Input: part model. Units: mm. Frame: model coordinates. A direction names the side the tool comes from. Coordinates: 2 decimals unless noted, no trailing zeros. Order: outer loops, then holes, each group sorted by start corner. A loop starts at its lowest first (then second) coordinate and runs counter-clockwise, first axis right, second up.
from build123d import *

# Parameters (mm, degrees)
F0_R          = 120
F1_DEPTH      = 12
F1_DEPTH_BACK = 38
F2_R          = 110
F2_R_2        = 17.5
F3_DEPTH      = 38
F4_R          = 5
F5_R          = 15.2795
F6_DEPTH      = 15.2795
F8_R          = 120
F9_DEPTH      = 5
F10_R         = 12.5
F11_DEPTH     = 55.001
F12_R         = 120
F12_R_2       = 110
F13_DEPTH     = 3
F14_W         = 5
F14_H         = 122.5
F14_W_2       = 122.5
F14_H_2       = 5
F15_DEPTH     = 3
F16_R         = 136.7884680592
F16_R_2       = 100.9393969777
F17_DEPTH     = 5
F19_R         = 4
F20_DEPTH     = 25
F22_R         = 4
F23_DEPTH     = 25


# Not quite as in the source:
# - a fillet or chamfer that OpenCascade refuses, or shapes differently, is made with other operations: its cross-section is extruded or revolved along the edge and cut away or added


with BuildPart() as f1:
    # F0 (on Top) → F1 (new body, two sides)
    with BuildSketch(Plane.XY) as f1_sk:
        Circle(F0_R)
    extrude(amount=F1_DEPTH)
    extrude(f1_sk.sketch, amount=-F1_DEPTH_BACK)

    # F2 (on face) → F3 (cut)
    with BuildSketch(Plane(origin=(0, 0, -38), x_dir=(1, 0, 0), z_dir=(0, 0, -1))):
        Circle(F2_R)
        Circle(F2_R_2, mode=Mode.SUBTRACT)
    extrude(amount=-F3_DEPTH, mode=Mode.SUBTRACT)

    # F4
    f4_edges = [f1.edges().sort_by_distance(p)[0] for p in [
        (-17.5, 0, 0),
        (-110, 0, 0),
    ]]
    fillet(f4_edges, radius=F4_R)

    # F5 (on face) → F6 (cut)
    with BuildSketch(Plane(origin=(0, 0, 0), x_dir=(1, 0, 0), z_dir=(0, 0, -1))):
        with Locations((-60, 60)):
            Circle(F5_R)
        with Locations((-60, -60)):
            Circle(F5_R)
        with Locations((60, -60)):
            Circle(F5_R)
        with Locations((60, 60)):
            Circle(F5_R)
    extrude(amount=-F6_DEPTH, mode=Mode.SUBTRACT)

    # F8 (on face) → F9 (join)
    with BuildSketch(Plane.XY.offset(12)):
        Circle(F8_R)
    extrude(amount=F9_DEPTH)

    # F10 (on face) → F11 (cut, through all)
    with BuildSketch(Plane(origin=(0, 0, -38), x_dir=(1, 0, 0), z_dir=(0, 0, -1))):
        Circle(F10_R)
    extrude(amount=-F11_DEPTH, mode=Mode.SUBTRACT)

    # F12 (on face) → F13 (cut)
    with BuildSketch(Plane.XY.offset(17)):
        Circle(F12_R)
        Circle(F12_R_2, mode=Mode.SUBTRACT)
    extrude(amount=-F13_DEPTH, mode=Mode.SUBTRACT)

    # F14 (on face) → F15 (cut)
    with BuildSketch(Plane.XY.offset(17)):
        with Locations((0, -63.75)):
            Rectangle(F14_W, F14_H)
        with Locations((-63.75, 0)):
            Rectangle(F14_W_2, F14_H_2)
        Rectangle(F14_W, F14_H_2)
        with Locations((63.75, 0)):
            Rectangle(F14_W_2, F14_H_2)
        with Locations((0, 63.75)):
            Rectangle(F14_W, F14_H)
    extrude(amount=-F15_DEPTH, mode=Mode.SUBTRACT)

    # F16 (on face) → F17 (cut)
    with BuildSketch(Plane(origin=(0, 0, -38), x_dir=(1, 0, 0), z_dir=(0, 0, -1))):
        Circle(F16_R)
        Circle(F16_R_2, mode=Mode.SUBTRACT)
    extrude(amount=-F17_DEPTH, mode=Mode.SUBTRACT)

    # F18: fillet of radius 15.2795 on 4 edges, made by hand

    # F18_s1 → F18_t2 (revolve)
    with BuildSketch(Plane.XZ.offset(60)):
        with BuildLine():
            ThreePointArc((75.2795, 0), (69.9309062658, 8.6278977111), (60.3560955627, 12))
            Line((60.3560955627, 12), (75.2795, 12))
            Line((75.2795, 12), (75.2795, 0))
        make_face()
    revolve(axis=Axis((60, -60, 12), (0, 0, -1)))

    # F18_s3 → F18_t4 (revolve)
    with BuildSketch(Plane.XZ.offset(60)):
        with BuildLine():
            ThreePointArc((-44.7205, 0), (-50.0690937342, 8.6278977111), (-59.6439044373, 12))
            Line((-59.6439044373, 12), (-44.7205, 12))
            Line((-44.7205, 12), (-44.7205, 0))
        make_face()
    revolve(axis=Axis((-60, -60, 12), (0, 0, -1)))

    # F18_s5 → F18_t6 (revolve)
    with BuildSketch(Plane.XZ.offset(-60)):
        with BuildLine():
            ThreePointArc((-44.7205, 0), (-50.0690937342, 8.6278977111), (-59.6439044373, 12))
            Line((-59.6439044373, 12), (-44.7205, 12))
            Line((-44.7205, 12), (-44.7205, 0))
        make_face()
    revolve(axis=Axis((-60, 60, 12), (0, 0, -1)))

    # F18_s7 → F18_t8 (revolve)
    with BuildSketch(Plane.XZ.offset(-60)):
        with BuildLine():
            ThreePointArc((75.2795, 0), (69.9309062658, 8.6278977111), (60.3560955627, 12))
            Line((60.3560955627, 12), (75.2795, 12))
            Line((75.2795, 12), (75.2795, 0))
        make_face()
    revolve(axis=Axis((60, 60, 12), (0, 0, -1)))

    # F19 (on offset) → F20 (cut)
    with BuildSketch(Plane.XZ.offset(120)):
        with Locations((0, -19)):
            Circle(F19_R)
    extrude(amount=-F20_DEPTH, mode=Mode.SUBTRACT)

    # F22 (on offset) → F23 (cut)
    with BuildSketch(Plane.XZ.offset(-120)):
        with Locations((0, -19)):
            Circle(F22_R)
    extrude(amount=F23_DEPTH, mode=Mode.SUBTRACT)


solid = f1.part
Item 1: Pin query (flat end, axial travel): pin 1 Ø1.5 at (y, z) = (-47, -21) entering from -X; pin 2 Ø1.5 at (x, z) = (-74, 15.5) entering from +Y; pin 3 Ø8 at (x, y) = (-36, 85) entering from -Z; pin 4 Ø15 at (x, y) = (0, 0) entering from -Z. Return the tip coordinate at first contact, or that it passes through.
Response values:
pin 1: stops at x = -110.73
pin 2: stops at y = 82.06
pin 3: stops at z = 0
pin 4: passes through
Item 2: Cut plane A-A on z = -26.5. Return loops of the section in (x, y).
Response values:
outline: circle Ø240 at (0, 0); circle Ø35 at (0, 0); hole circle Ø220 at (0, 0); hole circle Ø25 at (0, 0)
Item 3: Draft query along X for faces 1 (the face through (-1, -25, 0)), 2 (the face through (-45, -44, 17)), 3 (the face through (-0.521, -115.033, -15.034)), 4 (the face through (-78.608, -76.947, 15.521)). Return one class per face: pulls with the +X half, pulls with the -X half, needs draft (parallel to the pull), parting line crosses it, or undercut.
Response values:
face 1: undercut
face 2: needs draft
face 3: undercut
face 4: pulls with the -X half
Item 4: Access query for faces 5 (the face through (-23.846, 107.384, -19.196)), 6 (the face through (78.608, 76.947, 15.521)), 7 (the face through (-76.947, 78.608, 15.521)). Directions: +Z, -Z, +X, -X, +Y, -Y. A direction counts if a zero-diameter tool reaches every point of the face in a straight line with its end or side. Return the directions, or none.
Response values:
face 5: -Z
face 6: +Z, +X, +Y
face 7: +Z, -X, +Y
Item 5: Ray query, probe 1 along Y at (x, z) = (0, -11.25); probe 2 along Z at (x, y) = (0, 113.25). Return the intervals inside material, ascending.
Response values:
probe 1: y = -120 to -110, -17.5 to -12.5, 12.5 to 17.5, 110 to 120
probe 2: z = -33 to -23, -15 to 14
